from build123d import *

# Parameters (mm, degrees)
SKETCH1_R           = 3.175
SKETCH1_R_2         = 1.5
SKETCH1_R_3         = 3.5687
BOSS_EXTRUDE1_DEPTH = 12.7


with BuildPart() as part:
    # Sketch1 → Boss-Extrude1 (new body)
    with BuildSketch(Plane(origin=(0, 0, 0), x_dir=(1, 0, 0), z_dir=(0, 1, 0))):
        with BuildLine():
            Line((175, -200), (175, 200))
            ThreePointArc((175, 200), (0, 265.753645318), (-175, 200))
            Line((-175, 200), (-175, -200))
            ThreePointArc((-175, -200), (0, -265.753645318), (175, -200))
        make_face()
        with Locations((130.12, 112.41)):
            Circle(SKETCH1_R, mode=Mode.SUBTRACT)
        with Locations((130.12, 62.41)):
            Circle(SKETCH1_R, mode=Mode.SUBTRACT)
        with Locations((100.12, 112.41)):
            Circle(SKETCH1_R, mode=Mode.SUBTRACT)
        with Locations((100.12, 62.41)):
            Circle(SKETCH1_R, mode=Mode.SUBTRACT)
        with Locations((-130.12, 62.41)):
            Circle(SKETCH1_R, mode=Mode.SUBTRACT)
        with Locations((-100.12, 62.41)):
            Circle(SKETCH1_R, mode=Mode.SUBTRACT)
        with Locations((-100.12, 112.41)):
            Circle(SKETCH1_R, mode=Mode.SUBTRACT)
        with Locations((-130.12, 112.41)):
            Circle(SKETCH1_R, mode=Mode.SUBTRACT)
        with Locations((-130.12, -62.59)):
            Circle(SKETCH1_R, mode=Mode.SUBTRACT)
        with Locations((-100.12, -62.59)):
            Circle(SKETCH1_R, mode=Mode.SUBTRACT)
        with Locations((-100.12, -112.59)):
            Circle(SKETCH1_R, mode=Mode.SUBTRACT)
        with Locations((-130.12, -112.59)):
            Circle(SKETCH1_R, mode=Mode.SUBTRACT)
        with Locations((130.12, -62.59)):
            Circle(SKETCH1_R, mode=Mode.SUBTRACT)
        with Locations((100.12, -62.59)):
            Circle(SKETCH1_R, mode=Mode.SUBTRACT)
        with Locations((100.12, -112.59)):
            Circle(SKETCH1_R, mode=Mode.SUBTRACT)
        with Locations((130.12, -112.59)):
            Circle(SKETCH1_R, mode=Mode.SUBTRACT)
        with Locations((-99.51, 209.02)):
            Circle(SKETCH1_R_2, mode=Mode.SUBTRACT)
        with Locations((-60.265573644, 248.264426356)):
            Circle(SKETCH1_R_2, mode=Mode.SUBTRACT)
        with Locations((-27.75, 248.264426356)):
            Circle(SKETCH1_R_2, mode=Mode.SUBTRACT)
        with Locations((27.75, 248.264426356)):
            Circle(SKETCH1_R_2, mode=Mode.SUBTRACT)
        with Locations((60.265573644, 248.264426356)):
            Circle(SKETCH1_R_2, mode=Mode.SUBTRACT)
        with Locations((99.51, 209.02)):
            Circle(SKETCH1_R_2, mode=Mode.SUBTRACT)
        with Locations((-60.265573644, -248.264426356)):
            Circle(SKETCH1_R_2, mode=Mode.SUBTRACT)
        with Locations((99.51, -209.02)):
            Circle(SKETCH1_R_2, mode=Mode.SUBTRACT)
        with Locations((60.265573644, -248.264426356)):
            Circle(SKETCH1_R_2, mode=Mode.SUBTRACT)
        with Locations((-99.51, -209.02)):
            Circle(SKETCH1_R_2, mode=Mode.SUBTRACT)
        with Locations((-53.36, 168.6)):
            Circle(SKETCH1_R_2, mode=Mode.SUBTRACT)
        with Locations((50.74, 168.6)):
            Circle(SKETCH1_R_2, mode=Mode.SUBTRACT)
        with Locations((-53.36, 18.7)):
            Circle(SKETCH1_R_2, mode=Mode.SUBTRACT)
        with Locations((50.74, 18.7)):
            Circle(SKETCH1_R_2, mode=Mode.SUBTRACT)
        with Locations((50.74, -18.7)):
            Circle(SKETCH1_R_2, mode=Mode.SUBTRACT)
        with Locations((-53.36, -18.7)):
            Circle(SKETCH1_R_2, mode=Mode.SUBTRACT)
        with Locations((50.74, -168.6)):
            Circle(SKETCH1_R_2, mode=Mode.SUBTRACT)
        with Locations((-53.36, -168.6)):
            Circle(SKETCH1_R_2, mode=Mode.SUBTRACT)
        with Locations((-31, -204.574478526)):
            Circle(SKETCH1_R_2, mode=Mode.SUBTRACT)
        with Locations((-31, -254.574478526)):
            Circle(SKETCH1_R_2, mode=Mode.SUBTRACT)
        with Locations((31, -254.574478526)):
            Circle(SKETCH1_R_2, mode=Mode.SUBTRACT)
        with Locations((31, -204.574478526)):
            Circle(SKETCH1_R_2, mode=Mode.SUBTRACT)
        with Locations((-159.12, 0)):
            Circle(SKETCH1_R_3, mode=Mode.SUBTRACT)
        with Locations((-159.12, -180.95)):
            Circle(SKETCH1_R_3, mode=Mode.SUBTRACT)
        with Locations((-159.12, 187.3)):
            Circle(SKETCH1_R_3, mode=Mode.SUBTRACT)
        with Locations((159.12, -180.95)):
            Circle(SKETCH1_R_3, mode=Mode.SUBTRACT)
        with Locations((159.12, 0)):
            Circle(SKETCH1_R_3, mode=Mode.SUBTRACT)
        with Locations((159.12, 187.3)):
            Circle(SKETCH1_R_3, mode=Mode.SUBTRACT)
    extrude(amount=BOSS_EXTRUDE1_DEPTH)


solid = part.part
Input: part model. Units: mm. Frame: model coordinates. Coordinates: 2 decimals unless noted, no trailing zeros. Loops run counter-clockwise (first coordinate to the right, second up) from the corner with the lowest first, then second, coordinate; pieces in that order, holes last.
(1) Section A-A on x = 139. Return the cut outline in (y, z).
(2) Material intervals for probe 1 along X at (y, z) = (8.5, -62.41) (3 decimals); probe 2 along X at (y, z) = (3, -19); probe 3 along X at (y, z) = (5, 113), sorted ascending.
(3) Section B-B on y = 9.5. Count the separate pieces of the cut face and the enclosed holes in it, then the cut area to 3 significant figures.
Data:
1. outline: (0, -226.5) - (12.7, -226.5) - (12.7, 226.5) - (0, 226.5) - close
2. probe 1: x = -175 to -133.295, -126.945 to -103.295, -96.945 to 96.945, 103.295 to 126.945, 133.295 to 175
2. probe 2: x = -175 to -54.83, -51.89 to 49.27, 52.21 to 175
2. probe 3: x = -175 to -133.27, -126.97 to -103.27, -96.97 to 96.97, 103.27 to 126.97, 133.27 to 175
3. separate pieces: 1
3. enclosed holes: 44
3. area: 171,000 mm2
